```python
from build123d import *

# Parameters (mm, degrees)
SKETCH1_R           = 2.55
BOSS_EXTRUDE1_DEPTH = 4.8
BOSS_EXTRUDE2_DEPTH = 51.08
SKETCH3_R           = 19.05
BOSS_EXTRUDE3_DEPTH = 1.6
SKETCH4_R           = 3.175
BOSS_EXTRUDE8_DEPTH = 19.4


with BuildPart() as part:
    # Sketch1 → Boss-Extrude1 (new body)
    with BuildSketch(Plane.XY):
        with BuildLine():
            Line((-23.755, -28.2), (23.755, -28.2))
            ThreePointArc((23.755, -28.2), (26.898089642, -26.898089642), (28.2, -23.755))
            Line((28.2, -23.755), (28.2, 23.755))
            ThreePointArc((28.2, 23.755), (26.898089642, 26.898089642), (23.755, 28.2))
            Line((23.755, 28.2), (-23.755, 28.2))
            ThreePointArc((-23.755, 28.2), (-26.898089642, 26.898089642), (-28.2, 23.755))
            Line((-28.2, 23.755), (-28.2, -23.755))
            ThreePointArc((-28.2, -23.755), (-26.898089642, -26.898089642), (-23.755, -28.2))
        make_face()
        with Locations((-23.57, 23.57)):
            Circle(SKETCH1_R, mode=Mode.SUBTRACT)
        with Locations((23.57, 23.57)):
            Circle(SKETCH1_R, mode=Mode.SUBTRACT)
        with Locations((23.57, -23.57)):
            Circle(SKETCH1_R, mode=Mode.SUBTRACT)
        with Locations((-23.57, -23.57)):
            Circle(SKETCH1_R, mode=Mode.SUBTRACT)
    extrude(amount=BOSS_EXTRUDE1_DEPTH)

    # Sketch2 → Boss-Extrude2 (add)
    with BuildSketch(Plane(origin=(0, 0, 0), x_dir=(-1, 0, 0), z_dir=(0, 0, -1))):
        with BuildLine():
            Line((23.57, -18.94), (26.93, -18.94))
            ThreePointArc((26.93, -18.94), (27.828025612, -18.568025612), (28.2, -17.67))
            Line((28.2, -17.67), (28.2, 17.66630547))
            ThreePointArc((28.2, 17.66630547), (27.828025612, 18.564331082), (26.93, 18.93630547))
            Line((26.93, 18.93630547), (23.57, 18.93630547))
            ThreePointArc((23.57, 18.93630547), (20.293483176, 20.293483176), (18.93630547, 23.57))
            Line((18.93630547, 23.57), (18.93630547, 26.93))
            ThreePointArc((18.93630547, 26.93), (18.564331082, 27.828025612), (17.66630547, 28.2))
            Line((17.66630547, 28.2), (-17.67, 28.2))
            ThreePointArc((-17.67, 28.2), (-18.568025612, 27.828025612), (-18.94, 26.93))
            Line((-18.94, 26.93), (-18.94, 23.57))
            ThreePointArc((-18.94, 23.57), (-20.296095603, 20.296095603), (-23.57, 18.94))
            Line((-23.57, 18.94), (-26.93, 18.94))
            ThreePointArc((-26.93, 18.94), (-27.828025612, 18.568025612), (-28.2, 17.67))
            Line((-28.2, 17.67), (-28.2, -17.66630547))
            ThreePointArc((-28.2, -17.66630547), (-27.828025612, -18.564331082), (-26.93, -18.93630547))
            Line((-26.93, -18.93630547), (-23.57, -18.93630547))
            ThreePointArc((-23.57, -18.93630547), (-20.293483176, -20.293483176), (-18.93630547, -23.57))
            Line((-18.93630547, -23.57), (-18.93630547, -26.93))
            ThreePointArc((-18.93630547, -26.93), (-18.564331082, -27.828025612), (-17.66630547, -28.2))
            Line((-17.66630547, -28.2), (17.67, -28.2))
            ThreePointArc((17.67, -28.2), (18.568025612, -27.828025612), (18.94, -26.93))
            Line((18.94, -26.93), (18.94, -23.57))
            ThreePointArc((18.94, -23.57), (20.296095603, -20.296095603), (23.57, -18.94))
        make_face()
    extrude(amount=BOSS_EXTRUDE2_DEPTH)

    # Sketch3 → Boss-Extrude3 (add)
    with BuildSketch(Plane.XY.offset(4.8)):
        Circle(SKETCH3_R)
    extrude(amount=BOSS_EXTRUDE3_DEPTH)

    # Sketch4 → Boss-Extrude8 (add)
    with BuildSketch(Plane.XY.offset(6.4)):
        Circle(SKETCH4_R)
    extrude(amount=BOSS_EXTRUDE8_DEPTH)


solid = part.part
```
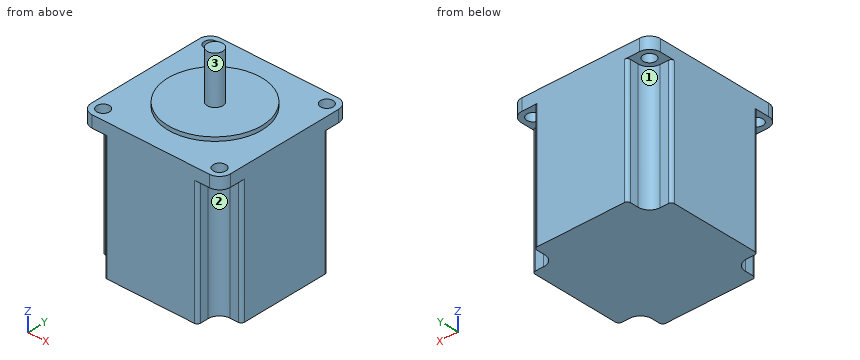
The model under review builds one solid part; all positions refer to its coordinate system, in mm. Face numbers are marked on the shaded views. A direction names the side the tool comes from. Coordinates: 2 decimals unless noted, no trailing zeros. Write each loop counter-clockwise with the first axis right and the second up, starting at its lowest first coordinate (ties: lowest second). Pieces come first, ordered by that corner, then holes.
1) Machinability: for the marked faces 1, 2 and 3, which of the approach directions +Z, -Z, +X, -X, +Y, -Y give a long, thin tool a straight path to every point of the face, cutting with its end or side? Answer none if there is none.
2) We need section A-A on y = 0. State the section outline as (x, z) points (3 decimals), then the cut area to 3 significant figures.
3) To check wall thickness, follow probe 1 along Y at (x, z) = (-23.57, 3.8); probe 2 along X at (y, z) = (-23, 1). State the ranges of each line that lie inside material, in increasing order.
4) We need section B-B on x = -22.5. State the section outline as (y, z) points, then the cut area to 3 significant figures.
5) Clearance check with flat-ended pins moving along their axes: pin 1 Ø1 at (x, z) = (-25, -38) entering from -Y; pin 2 Ø2.5 at (y, z) = (26, -21.5) entering from +X; pin 3 Ø1 at (x, y) = (-12, -0.5) entering from +Z; pin 4 Ø11.5 at (x, y) = (21, -24.5) entering from -Z. State where each tip first meets the part, or that it passes through.
6) We need section C-C on z = -2. State the section outline as (x, y) points.
Answer list:
1. face 1: -Z, -X, +Y
1. face 2: -Z, +X, -Y
1. face 3: +Z
2. outline: (-28.2, -51.08) - (28.2, -51.08) - (28.2, 4.8) - (19.05, 4.8) - (19.05, 6.4) - (3.175, 6.4) - (3.175, 25.8) - (-3.175, 25.8) - (-3.175, 6.4) - (-19.05, 6.4) - (-19.05, 4.8) - (-28.2, 4.8) - close
2. area: 3,340 mm2
3. probe 1: y = -28.2 to -26.12, -21.02 to 21.02, 26.12 to 28.2
3. probe 2: x = -28.2 to -26.06, -21.08 to 21.08, 26.06 to 28.2
4. outline: (-28.2, 0) - (-25.88, 0) - (-25.88, 4.8) - (-28.2, 4.8) - close; (-21.26, 0) - (-19.07, 0) - (-19.07, -51.08) - (19.06, -51.08) - (19.06, 0) - (21.26, 0) - (21.26, 4.8) - (-21.26, 4.8) - close; (25.88, 0) - (28.2, 0) - (28.2, 4.8) - (25.88, 4.8) - close
4. area: 2,170 mm2
5. pin 1: stops at y = -18.94
5. pin 2: stops at x = 18.94
5. pin 3: stops at z = 6.4
5. pin 4: stops at z = -51.08
6. outline: (-28.2, -17.67) arc R1.27 ccw to (-26.93, -18.94) - (-23.57, -18.94) arc R4.63 cw to (-18.94, -23.57) - (-18.94, -26.93) arc R1.27 ccw to (-17.67, -28.2) - (17.67, -28.2) arc R1.27 ccw to (18.94, -26.93) - (18.94, -23.57) arc R4.63 cw to (23.57, -18.94) - (26.93, -18.94) arc R1.27 ccw to (28.2, -17.67) - (28.2, 17.67) arc R1.27 ccw to (26.93, 18.94) - (23.57, 18.94) arc R4.63 cw to (18.94, 23.57) - (18.94, 26.93) arc R1.27 ccw to (17.67, 28.2) - (-17.67, 28.2) arc R1.27 ccw to (-18.94, 26.93) - (-18.94, 23.57) arc R4.63 cw to (-23.57, 18.94) - (-26.93, 18.94) arc R1.27 ccw to (-28.2, 17.67) - close
